Design review of the part built by this model. Coordinates are the model's own, in mm. Face numbers are marked on the shaded views. A direction names the side the tool comes from. Give positions to 0.01 mm unless a question says otherwise; leave off trailing zeros. Order: outer loops, then holes, each group sorted by start corner. A loop starts at its lowest first (then second) coordinate and runs counter-clockwise, first axis right, second up. Notation, with made-up numbers: M 83.25,-34.75 L 129.25,-34.75 A10 ccw 129.25,-30.75 Z; hole C 2,25.25 d1. An arc over 180 degrees is marked long. Answer as a JSON object with one key per item and string values.
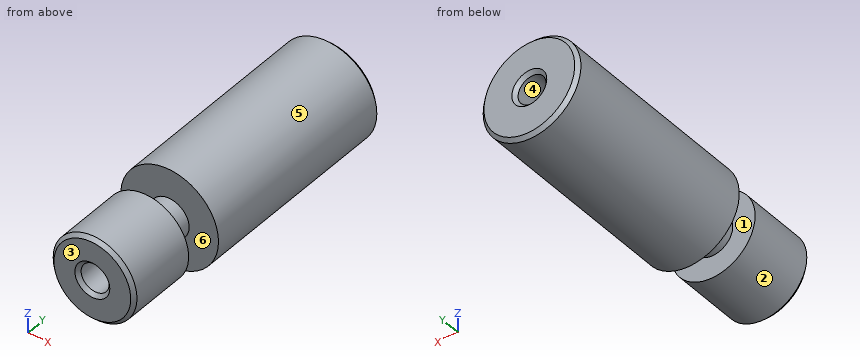
Autodesk Inventor part; units mm, degrees
ref_plane "YZ Plane" through (0, 0, 0) normal (1, 0, 0) x (0, 1, 0)
ref_plane "XZ Plane" through (0, 0, 0) normal (0, 1, 0) x (-1, 0, 0)
ref_plane "XY Plane" through (0, 0, 0) normal (0, 0, 1) x (1, 0, 0)
sketch "草圖1" plane through (0, 0, 0) normal (0, 1, 0) x (-1, 0, 0)
  circle A0 centre (0, 0) radius 3
  dimension "d0" = 6
extrude "擠出1" add sketch "草圖1" along normal blind 5
sketch "草圖2" plane through (0, 5, 0) normal (0, 1, 0) x (1, 0, 0)
  circle A0 centre (0, 0) radius 3
  circle A1 centre (0, 0) radius 1.4
  dimension "d4" = 2.8
extrude "擠出2" add sketch "草圖2" along normal blind 2.1 contours A1
sketch "草圖3" plane through (0, 7.1, 0) normal (0, 1, 0) x (1, 0, 0)
  circle A0 centre (0, 0) radius 1.4
  circle A1 centre (0, 0) radius 3.5
  dimension "d8" = 7
extrude "擠出3" add sketch "草圖3" along normal blind 14.8 contours A0 | A1
sketch "草圖5" plane through (0, 0, 0) normal (0, -1, 0) x (1, 0, 0)
  circle A0 centre (0, 0) radius 3
hole "孔1" at (0, 0, 0) direction (0, 1, 0) diameter 2 end through all
chamfer "倒角2" distance 0.25 angle 45 4 edges at (3, 0, 0) (0, 0, 1) (-3.5, 21.9, 0) (0, 21.9, 1)
thread "螺紋1"
thread "螺紋2"
properties part number "e3d_v6_heat_break"
(1) We need section D-D (y = 4.25). Write out the cut boundary in (x, z).
Checked values:
{"outline": "C 0,0 d6; hole C 0,0 d2"}
(2) We need section C-C (y = 15). Write out the cut boundary in (x, z).
Checked values:
{"outline": "C 0,0 d7; hole C 0,0 d2"}
(3) To check wall thickness, follow L1, parallel to X at y = 13.25, z = 0; L2, parallel to Y at x = 2.5, z = 0.5. State the ranges of each line that lie inside material, in increasing order. Write a range as from..to.
Checked values:
{"L1": "x = -3.5..-1, 1..3.5", "L2": "y = 0..5, 7.1..21.9"}
(4) We need section B-B (z = 0). Write out the cut boundary in (x, y).
Checked values:
{"outline": "M -3.5,7.1 L -1.4,7.1 L -1.4,5 L -3,5 L -3,0.25 L -2.75,0 L -1.25,0 L -1,0.25 L -1,21.65 L -1.25,21.9 L -3.25,21.9 L -3.5,21.65 Z; M 1,0.25 L 1.25,0 L 2.75,0 L 3,0.25 L 3,5 L 1.4,5 L 1.4,7.1 L 3.5,7.1 L 3.5,21.65 L 3.25,21.9 L 1.25,21.9 L 1,21.65 Z"}
(5) We need section A-A (x = 0). Write out the cut boundary in (y, z).
Checked values:
{"outline": "M 0,-2.75 L 0.25,-3 L 5,-3 L 5,-1.4 L 7.1,-1.4 L 7.1,-3.5 L 21.65,-3.5 L 21.9,-3.25 L 21.9,-1.25 L 21.65,-1 L 0.25,-1 L 0,-1.25 Z; M 0,1.25 L 0.25,1 L 21.65,1 L 21.9,1.25 L 21.9,3.25 L 21.65,3.5 L 7.1,3.5 L 7.1,1.4 L 5,1.4 L 5,3 L 0.25,3 L 0,2.75 Z"}
(6) Insertion check: pin 1 (4 mm diameter, centred on x = 3, y = 3.5, fed in from +Z). The pin has a flat end and moves straight along its axis. Give the tip position at first contact, or say it passes through.
Checked values:
{"pin 1": "stops at z = 2.83"}
(7) Draft analysis for pull direction X (two halves, no side actions). For the marked faces 4, 5 and 6, state which applies: +X half, -X half, draft (parallel to the pull), parting line (faces both ways), or undercut.
Checked values:
{"face 4": "undercut", "face 5": "parting line", "face 6": "draft"}
(8) Tool access review of the marked faces 1, 2 and 3: name each direction out of +Z, -Z, +X, -X, +Y, -Y from which nothing blocks a thin tool from reaching the whole face with its end or side.
Checked values:
{"face 1": "none", "face 2": "-Y", "face 3": "+Z, -Z, +X, -X, -Y"}
